Design review of the part built by this model. Coordinates are the model's own, in mm. Coordinates: 2 decimals unless noted, no trailing zeros. Order: outer loops, then holes, each group sorted by start corner. A loop starts at its lowest first (then second) coordinate and runs counter-clockwise, first axis right, second up. Notation, with made-up numbers: (-7.5, 41) - (0.5, 41) arc R18 cw to (0.5, 52) - close; hole circle Ø2 at (71.5, 19). An arc over 180 degrees is marked (long way). Write item = value, one per line. Start each with the question number.
```python
from build123d import *

# Parameters (mm, degrees)
F1_DEPTH = 25.4
F2_R     = 18.728572
F3_DEPTH = 25.4


with BuildPart() as f1:
    # F0 (on Front) → F1 (new body)
    with BuildSketch(Plane.XZ):
        Polygon((-89.339584, -8.090763), (0, -4.123797), (25.28479, -3.994782), (33.038791, 54.881528), (-78.551404, 47.953002), align=None)
    extrude(amount=F1_DEPTH)

    # F2 (on face) → F3 (cut)
    with BuildSketch(Plane(origin=(0, 0, 0), x_dir=(-1, 0, 0), z_dir=(0, 1, 0))):
        with Locations((37.289418, 17.826317)):
            Circle(F2_R)
    extrude(amount=-F3_DEPTH, mode=Mode.SUBTRACT)


solid = f1.part
```
Item 1: For P1, Ø3, axis at x = -31.5, y = -22, coming from the -Z side; P2, Ø12, axis at x = -30.5, z = 19.5, coming from the +Y side; P3, Ø8, axis at y = -5, z = 14.5, coming from the -X side; P4, Ø5, axis at x = -25, y = -13.5, coming from the +Z side, all flat-tipped, find the tip position at first contact; note any pin that passes through.
Item 2: For line 1 (X direction, y = -19.75, z = 25); line 2 (X direction, y = -5, z = 3); line 3 (Z direction, x = -43, y = -11), list the stretches that pass through material, from the lowest coordinate up.
Item 3: Add section B-B on x = -50. Give the boundary of the cut face in (y, z), plus the area to 3 significant figures.
Item 4: Add section C-C on y = -14.5. Give the boundary of the cut face in (x, z), plus the area to 3 significant figures.
Item 5: Add section A-A on z = 33.5. Give the boundary of the cut face in (x, y).
Item 6: Mouldability with a two-part tool opening along X and no side actions: class faces 1 (the flat face through (-21.975, -12.522, 51.466)), 2 (the cylindrical face through (-45.93, -12.52, 1.21)), 3 (the flat face through (-15, 0, 24)), 4 (the flat face through (-45.295, -12.522, -6.135)) as +X half, -X half, draft (parallel to the pull), parting line (faces both ways), or undercut.
Item 7: Add section D-D on z = 44.5. Give the boundary of the cut face in (x, y), plus the area to 3 significant figures.
Worked out:
q1.P1 = -5.59
q1.P2 = through
q1.P3 = -85.76
q1.P4 = 51.43
q2.line_1 = -82.97 to -54.59, -19.99 to 29.1
q2.line_2 = -87.2 to -48.73, -25.85 to 26.21
q2.line_3 = -6.03 to -0.01, 35.66 to 50.16
q3.outline = (-25.4, -6.34) - (0, -6.34) - (0, 4.07) - (-25.4, 4.07) - close; (-25.4, 31.58) - (0, 31.58) - (0, 49.73) - (-25.4, 49.73) - close
q3.area = 725 mm2
q4.outline = (-89.34, -8.09) - (0, -4.12) - (25.28, -3.99) - (33.04, 54.88) - (-78.55, 47.95) - close; hole circle Ø37.46 at (-37.29, 17.83)
q4.area = 5,300 mm2
q5.outline = (-81.33, -25.4) - (-47.54, -25.4) - (-47.54, 0) - (-81.33, 0) - close; (-27.04, -25.4) - (30.22, -25.4) - (30.22, 0) - (-27.04, 0) - close
q6.face_1 = -X half
q6.face_2 = undercut
q6.face_3 = draft
q6.face_4 = +X half
q7.outline = (-79.22, -25.4) - (31.67, -25.4) - (31.67, 0) - (-79.22, 0) - close
q7.area = 2,820 mm2
